Geometry: final body of the model. Coordinates: model frame, mm. A direction names the side the tool comes from. Give positions to 0.01 mm unless a question says otherwise; leave off trailing zeros. Loops run counter-clockwise (first coordinate to the right, second up) from the corner with the lowest first, then second, coordinate; pieces in that order, holes last.
```python
from build123d import *

# Parameters (mm, degrees)
SKETCH_1_R          = 2.5
EXTRUDE_1_DEPTH     = 3
SKETCH_2_R          = 1.5
EXTRUDE_2_DEPTH     = 20
CUT_EXTRUDE_1_DEPTH = 1.65


with BuildPart() as part:
    # 草图1 → 凸台-拉伸1 (new body)
    with BuildSketch(Plane(origin=(0, 0, 0), x_dir=(1, 0, 0), z_dir=(0, 1, 0))):
        Circle(SKETCH_1_R)
    extrude(amount=EXTRUDE_1_DEPTH)

    # 草图2 → 凸台-拉伸2 (add)
    with BuildSketch(Plane(origin=(0, 3, 0), x_dir=(1, 0, 0), z_dir=(0, 1, 0))):
        Circle(SKETCH_2_R)
    extrude(amount=EXTRUDE_2_DEPTH)

    # 草图3 → 切除-拉伸1 (cut)
    with BuildSketch(Plane.XZ):
        Polygon((1.425, 0), (0.7125, 1.2340862), (-0.7125, 1.2340862), (-1.425, 0), (-0.7125, -1.2340862), (0.7125, -1.2340862), align=None)
    extrude(amount=-CUT_EXTRUDE_1_DEPTH, mode=Mode.SUBTRACT)


solid = part.part
```
Q1. Section query B-B, the plane z = 0.3. Return loops of the section in (x, y), and give its area (3 significant figures).
Q2. Section query C-C, the plane y = 15. Return loops of the section in (x, z), and give its area (3 significant figures).
Q3. Material intervals for probe 1 along Y at (x, z) = (0, -2.3); probe 2 along Y at (x, z) = (-0.3, -0.65); probe 3 along Z at (x, y) = (-0.45, 4.5), sorted ascending.
Q4. Pin query (flat end, axial travel): pin 1 Ø1.5 at (y, z) = (12, 1) entering from +X; pin 2 Ø2 at (x, y) = (0.5, 5.5) entering from -Z; pin 3 Ø2 at (x, z) = (-1, 0.5) entering from -Y; pin 4 Ø1 at (x, z) = (-1.5, 1.5) entering from +Y. Return the tip coordinate at first contact, or that it passes through.
Q5. Mould query, pull axis X, two halves, no side actions, for faces 4 (the face through (0, 3, 2)), 5 (the face through (0, 1, -1.234)), 6 (the face through (-0.54, 1.48, 2.44)). Classes: +X half, -X half, draft (parallel to the pull), parting line (faces both ways), or undercut.
Q6. Section query D-D, the plane x = -1.75. Return loops of the section in (y, z).
Q7. Reachability of faces 1 (the face through (-1.5, 12.86, -0.07)), 2 (the face through (0, 1, 1.234)), 3 (the face through (0, 23, 0)) from +Z, -Z, +X, -X, +Y, -Y: full face, straight path, thin tool, end or side. Return the list, or none.
Q8. Section query A-A, the plane x = 0. Return loops of the section in (y, z), and give its area (3 significant figures).
Resolved:
1. outline: (-2.48, 0) - (-1.25, 0) - (-1.25, 1.65) - (1.25, 1.65) - (1.25, 0) - (2.48, 0) - (2.48, 3) - (1.47, 3) - (1.47, 23) - (-1.47, 23) - (-1.47, 3) - (-2.48, 3) - close
1. area: 69.5 mm2
2. outline: circle Ø3 at (0, 0)
2. area: 7.07 mm2
3. probe 1: y = 0 to 3
3. probe 2: y = 1.65 to 23
3. probe 3: z = -1.43 to 1.43
4. pin 1: stops at x = 1.48
4. pin 2: stops at z = -1.5
4. pin 3: stops at y = 0
4. pin 4: stops at y = 3
5. face 4: draft
5. face 5: undercut
5. face 6: parting line
6. outline: (0, -1.79) - (3, -1.79) - (3, 1.79) - (0, 1.79) - close
7. face 1: +Y
7. face 2: -Y
7. face 3: +Z, -Z, +X, -X, +Y
8. outline: (0, -2.5) - (3, -2.5) - (3, -1.5) - (23, -1.5) - (23, 1.5) - (3, 1.5) - (3, 2.5) - (0, 2.5) - (0, 1.23) - (1.65, 1.23) - (1.65, -1.23) - (0, -1.23) - close
8. area: 70.9 mm2
